Check sheet for the drawn part. Datum: minimum x, y, z corner. Units: mm. A direction names the side the tool comes from. Give positions to 0.01 mm unless a question says otherwise; leave off trailing zeros. Loops run counter-clockwise (first coordinate to the right, second up) from the corner with the lowest first, then second, coordinate; pieces in that order, holes last.
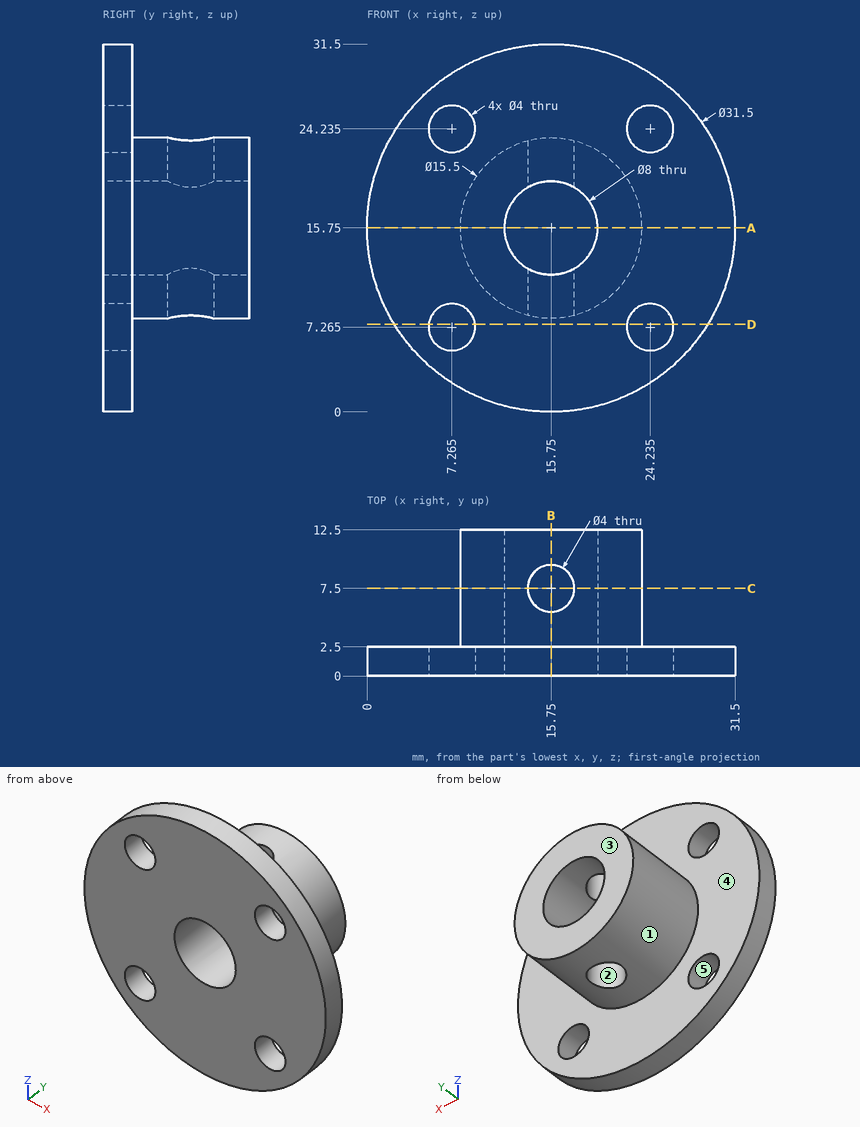
(1) Section check B-B on x = 15.75. Record the boundary of the cut face in (y, z).
(2) Section check A-A on z = 15.75. Record the boundary of the cut face in (x, y), plus the area to 3 significant figures.
(3) Material ranges on line 1 (X direction, y = 5.5, z = 15.5); line 2 (Y direction, x = 15.75, z = 10.7); line 3 (Z direction, x = 25, y = 2), recorded low to high.
(4) Gauge pin test, flat ends, axial feed: pin 1 Ø1.5 at (x, y) = (21.5, 10) entering from -Z; pin 2 Ø3.5 at (x, z) = (24.24, 24.24) entering from -Y; pin 3 Ø2 at (y, z) = (4, 18) entering from +X; pin 4 Ø3 at (x, y) = (19, 1.5) entering from -Z. Record the tip position at first contact, or that the pin passes through.
(5) Access from +Z, -Z, +X, -X, +Y, -Y to the whole of each face (thin tool, end or side, straight path). Record for the marked faces 4 and 5.
(6) Section check C-C on y = 7.5. Record the boundary of the cut face in (x, z), plus the area to 3 significant figures.
(7) Section check D-D on z = 7.5. Record the boundary of the cut face in (x, y).
(8) Release check for a two-part mould opening along X. For the marked faces 1, 2 and 3 record: pulls with the +X half, pulls with the -X half, needs draft (parallel to the pull), parting line crosses it, or undercut.
Computed values:
1. outline: (0, 0) - (2.5, 0) - (2.5, 8) - (5.5, 8) - (5.5, 11.75) - (0, 11.75) - close; (0, 19.75) - (5.5, 19.75) - (5.5, 23.5) - (2.5, 23.5) - (2.5, 31.5) - (0, 31.5) - close; (9.5, 8) - (12.5, 8) - (12.5, 11.75) - (9.5, 11.75) - close; (9.5, 19.75) - (12.5, 19.75) - (12.5, 23.5) - (9.5, 23.5) - close
2. outline: (0, 0) - (11.75, 0) - (11.75, 12.5) - (8, 12.5) - (8, 2.5) - (0, 2.5) - close; (19.75, 0) - (31.5, 0) - (31.5, 2.5) - (23.5, 2.5) - (23.5, 12.5) - (19.75, 12.5) - close
2. area: 134 mm2
3. line 1: x = 8 to 11.76, 19.74 to 23.5
3. line 2: y = 0 to 5.5, 9.5 to 12.5
3. line 3: z = 3 to 5.42, 9.11 to 22.39, 26.08 to 28.5
4. pin 1: stops at z = 9.83
4. pin 2: passes through
4. pin 3: stops at x = 23.4
4. pin 4: stops at z = 0.1
5. face 4: +Y
5. face 5: +Y, -Y
6. outline: (13.75, 8.26) - (13.75, 12.29) arc R4 cw to (13.75, 19.21) - (13.75, 23.24) arc R7.75 ccw to start; (17.75, 8.26) arc R7.75 ccw to (17.75, 23.24) - (17.75, 19.21) arc R4 cw to (17.75, 12.29) - close
6. area: 108 mm2
7. outline: (2.33, 0) - (5.28, 0) - (5.28, 2.5) - (2.33, 2.5) - close; (9.25, 0) - (22.25, 0) - (22.25, 2.5) - (9.25, 2.5) - close; (26.22, 0) - (29.17, 0) - (29.17, 2.5) - (26.22, 2.5) - close
8. face 1: parting line crosses it
8. face 2: undercut
8. face 3: needs draft
